Read the model definition and answer for the solid it produces. Units are mm, in the model's axes. Face numbers are marked on the shaded views. A direction names the side the tool comes from. Coordinates: 2 decimals unless noted, no trailing zeros. Write each loop counter-clockwise with the first axis right and the second up, starting at its lowest first coordinate (ties: lowest second). Pieces come first, ordered by that corner, then holes. Notation, with made-up numbers: (-38, 42.5) -> (4, 42.5) arc R31 cw to (4, 78.5) -> close; hole circle Ø10 at (49.25, -17.75). An arc over 180 degrees is marked (long way). Answer as a JSON object with one key per item and string values. Group by question number.
(1) Find section A-A (z = -7.5). Give the vertices of the cut face in (x, y).
(2) Which of the six approach directions +Z, -Z, +X, -X, +Y, -Y give full straight-line access (tool end or side, diameter ignored) to the marked faces 3 and 4?
(3) Straight lines are drawn through the part: L1, parallel to X at y = 32, z = -7.5; L2, parallel to X at y = 30.25, z = -8; L3, parallel to Z at x = -22.5, y = 33. For each, find the intervals that lie inside material, in ascending order.
(4) For a pull along X with two mould halves and no side action, classify the marked faces 1 and 2 as +X half, -X half, draft (parallel to the pull), parting line (faces both ways), or undercut.
(5) Flat-ended cylindrical pins translate along their axes: P1, Ø8, axis at x = -25, y = 38.5, coming from the -Z side; P2, Ø3, axis at x = -43.5, y = 35.5, coming from the -Z side; P3, Ø8, axis at y = 26, z = 1, coming from the +X side; P4, Ø2, axis at y = 28.5, z = -5.5, coming from the +X side. Find the tip coordinate at first contact, or state that the pin passes through.
from build123d import *

# Parameters (mm, degrees)
F0_R     = 6
F1_DEPTH = 7.5
F2_DEPTH = 10
F3_R     = 7.49999


# Not quite as in the source:
# - a fillet or chamfer is up to 0.001 mm smaller than in the source, because OpenCascade refuses the exact size


with BuildPart() as f1:
    # F0 (on Top) → F1 (new body)
    with BuildSketch(Plane.XY):
        with BuildLine():
            Line((-17.8126084931, 40.3974354923), (-53.2126084931, 40.3974354923))
            ThreePointArc((-53.2126084931, 40.3974354923), (-59.2583714722, 37.8931984714), (-61.7626084931, 31.8474354923))
            ThreePointArc((-61.7626084931, 31.8474354923), (-59.2583714722, 25.8016725131), (-53.2126084931, 23.2974354923))
            Line((-53.2126084931, 23.2974354923), (-17.8126084931, 23.2974354923))
            ThreePointArc((-17.8126084931, 23.2974354923), (-11.7668455139, 25.8016725131), (-9.2626084931, 31.8474354923))
            ThreePointArc((-9.2626084931, 31.8474354923), (-11.7668455139, 37.8931984714), (-17.8126084931, 40.3974354923))
        make_face()
        with Locations((-53.2126084931, 31.8474354923)):
            Circle(F0_R, mode=Mode.SUBTRACT)
        with Locations((-35.5126084931, 31.8474354923)):
            Circle(F0_R, mode=Mode.SUBTRACT)
        with Locations((-17.8126084931, 31.8474354923)):
            Circle(F0_R, mode=Mode.SUBTRACT)
        with Locations((-53.2126084931, 31.8474354923)):
            Circle(F0_R)
        with Locations((-35.5126084931, 31.8474354923)):
            Circle(F0_R)
        with Locations((-17.8126084931, 31.8474354923)):
            Circle(F0_R)
    extrude(amount=F1_DEPTH)

    # F0 (on Top) → F2 (join)
    with BuildSketch(Plane.XY):
        with Locations((-53.2126084931, 31.8474354923)):
            Circle(F0_R)
        with Locations((-35.5126084931, 31.8474354923)):
            Circle(F0_R)
        with Locations((-17.8126084931, 31.8474354923)):
            Circle(F0_R)
    extrude(amount=-F2_DEPTH)

    # F3 (radius 7.5 in the source; OpenCascade refuses exactly that, so slightly less here)
    f3_edges = [f1.edges().sort_by_distance(p)[0] for p in [
        (-61.762608, 31.847435, 7.5),
    ]]
    fillet(f3_edges, radius=F3_R)


solid = f1.part
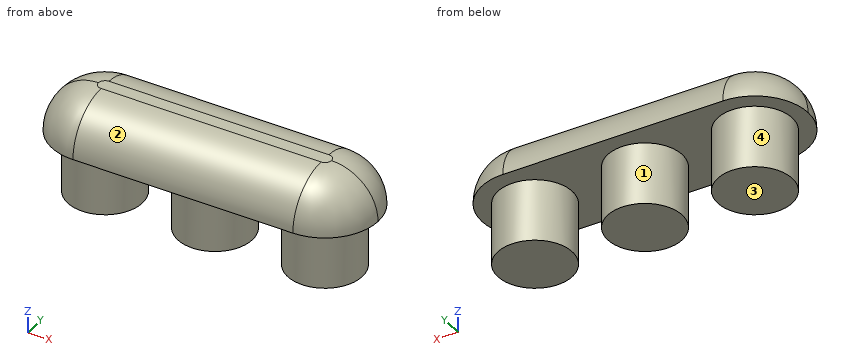
Results below:
{
 "1": {"outline": "circle Ø12 at (-53.21, 31.85); circle Ø12 at (-35.51, 31.85); circle Ø12 at (-17.81, 31.85)"},
 "2": {"face 3": "-Z, +X, -X, +Y, -Y", "face 4": "-Z"},
 "3": {"L1": "x = -59.21 to -47.21, -41.51 to -29.51, -23.81 to -11.81", "L2": "x = -59 to -47.43, -41.3 to -29.73, -23.6 to -12.03", "L3": "z = -10 to 7.5"},
 "4": {"face 1": "undercut", "face 2": "draft"},
 "5": {"P1": "stops at z = -10", "P2": "stops at z = 0", "P3": "stops at x = -9.48", "P4": "stops at x = -12.29"}
}
